Input: part model. Units: mm. Frame: model coordinates. A direction names the side the tool comes from. Round coordinates to 2 decimals unless told otherwise and drop trailing zeros. Write each loop counter-clockwise with the first axis right and the second up, starting at its lowest first coordinate (ties: lowest second). Pieces come first, ordered by that corner, then holes. Notation, with made-up numbers: (9, 20) -> (19, 20) arc R30 cw to (19, 50) -> close; hole circle Ø3 at (-35, 4.25). An arc over 180 degrees is marked (long way). Use CSV: the item, a comma, the result in double quotes.
```python
from build123d import *

# Parameters (mm, degrees)
SKETCH1_R           = 7.62
SKETCH1_W           = 12.7
SKETCH1_H           = 6.35
BOSS_EXTRUDE1_DEPTH = 25.4
BOSS_EXTRUDE2_DEPTH = 3.175
CUT_EXTRUDE1_REACH  = 35.02
SKETCH4_R           = 1.0414


with BuildPart() as part:
    # Sketch1 → Boss-Extrude1 (new body)
    with BuildSketch(Plane(origin=(0, 0, 0), x_dir=(1, 0, 0), z_dir=(0, 1, 0))):
        with BuildLine():
            Line((-9.525, -22.225), (9.525, -22.225))
            Line((9.525, -22.225), (9.525, -5.08))
            ThreePointArc((9.525, -5.08), (0, 10.795), (-9.525, -5.08))
            Line((-9.525, -5.08), (-9.525, -22.225))
        make_face()
        Circle(SKETCH1_R, mode=Mode.SUBTRACT)
        with Locations((0, -15.875)):
            Rectangle(SKETCH1_W, SKETCH1_H, mode=Mode.SUBTRACT)
    extrude(amount=BOSS_EXTRUDE1_DEPTH)

    # Sketch3 → Boss-Extrude2 (add)
    with BuildSketch(Plane(origin=(0, 0, 15.875), x_dir=(-1, 0, 0), z_dir=(0, 0, -1))):
        Polygon((-9.525, 22.225), (-9.525, 15.875), (-15.875, 19.05), (-15.875, 25.4), (-12.7, 25.4), (-12.7, 22.225), align=None)
    boss_extrude2 = extrude(amount=BOSS_EXTRUDE2_DEPTH)

    # Mirror1: Boss-Extrude2 across plane
    add(boss_extrude2.mirror(Plane(origin=(0, 0, 0), x_dir=(0, 0, 1), z_dir=(1, 0, 0))))

    # Sketch4 → Cut-Extrude1 (cut, up to next)
    with BuildSketch(Plane(origin=(0, 0, -10.795), x_dir=(-1, 0, 0), z_dir=(0, 0, -1)), mode=Mode.PRIVATE) as cut_extrude1_sk1:
        with Locations((0, 8.382)):
            Circle(SKETCH4_R)
    cut_extrude1_tool1 = extrude(cut_extrude1_sk1.sketch, amount=-CUT_EXTRUDE1_REACH, mode=Mode.PRIVATE) & part.part
    add(cut_extrude1_tool1.solids().sort_by_distance((0, 8.382, -10.795))[0], mode=Mode.SUBTRACT)
    # Sketch4 → Cut-Extrude1 (cut, up to next)
    with BuildSketch(Plane(origin=(0, 0, -10.795), x_dir=(-1, 0, 0), z_dir=(0, 0, -1)), mode=Mode.PRIVATE) as cut_extrude1_sk2:
        with Locations((0, 17.018)):
            Circle(SKETCH4_R)
    cut_extrude1_tool2 = extrude(cut_extrude1_sk2.sketch, amount=-CUT_EXTRUDE1_REACH, mode=Mode.PRIVATE) & part.part
    add(cut_extrude1_tool2.solids().sort_by_distance((0, 17.018, -10.795))[0], mode=Mode.SUBTRACT)


solid = part.part
```
Item 1: Pull-direction query (Z, two-part tool) for faces 5 (the face through (-13, 21, 15.875)), 6 (the face through (6.35, 13, 16)), 7 (the face through (-11, 22.225, 14)); classes: +Z half, -Z half, draft (parallel to the pull), parting line (faces both ways), or undercut.
Worked answers:
face 5,"+Z half"
face 6,"undercut"
face 7,"draft"
Item 2: Section query D-D on x = -2.5. Return the cut outline in (y, z) (3 decimals), plus the area to 3 significant figures.
Worked answers:
outline,"(0, -10.502) -> (25.4, -10.502) -> (25.4, -7.198) -> (0, -7.198) -> close; (0, 7.198) -> (25.4, 7.198) -> (25.4, 12.7) -> (0, 12.7) -> close; (0, 19.05) -> (25.4, 19.05) -> (25.4, 22.225) -> (0, 22.225) -> close"
area,"304 mm²"
Item 3: Set-up query: faces 1 (the face through (12.656, 17.44, 14.31)), 2 (the face through (0.226, 7.365, -9.193)), 3 (the face through (13, 21, 12.7)), 4 (the face through (-13, 21, 12.7)). Return all of +Z, -Z, +X, -X, +Y, -Y with unobstructed straight access to the full face (end or side cutting, diameter ignored); none if empty.
Worked answers:
face 1,"+Z, +X, -Y"
face 2,"-Z"
face 3,"+X, +Y, -Y"
face 4,"-X, +Y, -Y"
Item 4: First-contact query: pin 1 Ø1.6 at (x, z) = (-11, 14) entering from +Y (3 decimals); pin 2 Ø4 at (y, z) = (12.5, -5) entering from -X; pin 3 Ø5 at (y, z) = (12, 10.5) entering from +X (3 decimals). Flat tips, straight axial feed; report the tip coordinate or a pass-through.
Worked answers:
pin 1,"stops at y = 22.225"
pin 2,"stops at x = -10.37"
pin 3,"stops at x = 9.525"
Item 5: Section query C-C on x = 3. Return the cut outline in (y, z) (3 decimals), plus the area to 3 significant figures.
Worked answers:
outline,"(0, -10.37) -> (25.4, -10.37) -> (25.4, -7.005) -> (0, -7.005) -> close; (0, 7.005) -> (25.4, 7.005) -> (25.4, 12.7) -> (0, 12.7) -> close; (0, 19.05) -> (25.4, 19.05) -> (25.4, 22.225) -> (0, 22.225) -> close"
area,"311 mm²"
Item 6: Section query A-A on y = 11.75. Return the cut outline in (x, z) (3 decimals), plus the area to 3 significant figures.
Worked answers:
outline,"(-9.525, 5.08) arc R10.795 ccw (long way) to (9.525, 5.08) -> (9.525, 22.225) -> (-9.525, 22.225) -> close; hole circle Ø15.24 at (0, 0); hole (-6.35, 12.7) -> (6.35, 12.7) -> (6.35, 19.05) -> (-6.35, 19.05) -> close"
area,"352 mm²"
Item 7: Section query B-B on z = 0. Return the cut outline in (x, y) (3 decimals), plus the area to 3 significant figures.
Worked answers:
outline,"(-10.795, 0) -> (-7.62, 0) -> (-7.62, 25.4) -> (-10.795, 25.4) -> close; (7.62, 0) -> (10.795, 0) -> (10.795, 25.4) -> (7.62, 25.4) -> close"
area,"161 mm²"
Item 8: Line query: line 1 (Y direction, x = 0, z = -8.3); line 2 (Z direction, x = -0.5, y = 13) (3 decimals); line 3 (Z direction, x = 6, y = 21.25) (3 decimals). Output: solid intervals per line, ascending.
Worked answers:
line 1,"y = 0 to 7.34, 9.42 to 15.98, 18.06 to 25.4"
line 2,"z = -10.783 to -7.604, 7.604 to 12.7, 19.05 to 22.225"
line 3,"z = -8.974 to -4.697, 4.697 to 12.7, 19.05 to 22.225"
